Build history of the part. All positions in model axes, mm. A direction names the side the tool comes from. Round coordinates to 2 decimals unless told otherwise and drop trailing zeros. Write each loop counter-clockwise with the first axis right and the second up, starting at its lowest first coordinate (ties: lowest second). Pieces come first, ordered by that corner, then holes. Notation, with made-up numbers: M -4.75,47 L 36.25,47 A15 ccw 36.25,68 Z; hole C 16.5,19 d8. An arc over 180 degrees is marked long. Write item = value, one per line. Start each with the question number.
Q1. Band-saw the part on D-D on y = 0. Write the cut outline in (x, z), plus the area to 3 significant figures.
Q2. Band-saw the part on B-B on y = 9.75. Write the cut outline in (x, z), plus the area to 3 significant figures.
Q3. Tool access for faces 1 (the flat face through (0, 0, 70.202)), 2 (the cylindrical face through (0, -12, 62)), 3 (the flat face through (0, 0, 77.202)): list every direction of +Z, -Z, +X, -X, +Y, -Y with a clear straight run to the whole face (end or side of a thin tool).
Q4. Drop flat-ended pins along their axis: P1, Ø13, axis at y = -2, z = 65, coming from the +X side; P2, Ø7.5, axis at x = -7.5, y = -2, coming from the -Z side; P3, Ø2, axis at x = 10, y = 3, coming from the -Z side; P4, Ø3, axis at x = -2.5, z = 59, coming from the +Y side. Give the stop position or say it passes through.
Q5. Band-saw the part on A-A on z = 59. Write the cut outline in (x, y), plus the area to 3 significant figures.
Q6. Band-saw the part on C-C on x = 0. Write the cut outline in (y, z).
Q7. Pull direction Z, two halves, no side cores. Call faces 4 (the flat face through (8, 0, 74.202)), 5 (the cylindrical face through (0, 12, 62)), 6 (the flat face through (-5, 0, 71)): released by +Z, released by -Z, zero draft, split by the parting line, or undercut.
Q8. Probe L1, parallel to Z at x = 0, y = 7.5; L2, parallel to X at y = -4, z = 70.5; L3, parallel to Y at x = 0, z = 65.5. List the from-to ranges inside material, lowest first.
```python
from build123d import *

# Parameters (mm, degrees)
F1_W          = 15
F1_H          = 25
F3_T          = -3
F4_DEPTH      = 12.0000001006
F4_DEPTH_BACK = 12.0000001006
F5_R          = 2.5
F6_DEPTH      = 5
F7_W          = 10
F7_H          = 7
F8_DEPTH      = 12
F8_DEPTH_BACK = 12


with BuildPart() as f2:
    # F1 (on Front) → F2 (revolve)
    with BuildSketch(Plane.XZ):
        with Locations((7.5, 64.7015325446)):
            Rectangle(F1_W, F1_H)
    revolve(axis=Axis((0, 0, 62.2015325446), (0, 0, 1)))

    # F3
    f3_openings = [f2.faces().sort_by_distance(p)[0] for p in [
        (0, 0, 52.201533),
    ]]
    offset(amount=F3_T, openings=f3_openings)

    # F0 (on Front) → F4 (join, two sides)
    with BuildSketch(Plane.XZ) as f4_sk:
        with BuildLine():
            ThreePointArc((-5, 62.2015325446), (-4.0541927813, 59.2751831307), (-1.5745916432, 57.4559386769))
            ThreePointArc((-1.5745916432, 57.4559386769), (2.9263494138, 58.1473397632), (5, 62.2015325446))
            Line((5, 62.2015325446), (5, 70.2015325446))
            Line((5, 70.2015325446), (-5, 70.2015325446))
            Line((-5, 70.2015325446), (-5, 62.2015325446))
        make_face()
        with BuildLine():
            ThreePointArc((2.5, 62.2015325446), (1.4631747069, 60.1744361539), (-0.7872958216, 59.8287356107))
            ThreePointArc((-0.7872958216, 59.8287356107), (-1.4631747069, 64.2286289352), (2.5, 62.2015325446))
        make_face(mode=Mode.SUBTRACT)
    extrude(amount=-F4_DEPTH)
    extrude(f4_sk.sketch, amount=F4_DEPTH_BACK)

    # F5 (on Front) → F6 (cut, symmetric)
    with BuildSketch(Plane.XZ):
        with BuildLine():
            Line((5, 70.2015325446), (-5, 70.2015325446))
            Line((-5, 70.2015325446), (-5, 62.2015325446))
            ThreePointArc((-5, 62.2015325446), (0, 57.2015325446), (5, 62.2015325446))
            Line((5, 62.2015325446), (5, 70.2015325446))
        make_face()
        with Locations((0, 62.2015325446)):
            Circle(F5_R, mode=Mode.SUBTRACT)
    extrude(amount=F6_DEPTH, both=True, mode=Mode.SUBTRACT)

    # F7 (on Front) → F8 (join, two sides)
    with BuildSketch(Plane.XZ) as f8_sk:
        with Locations((0, 73.7015325446)):
            Rectangle(F7_W, F7_H)
    extrude(amount=F8_DEPTH)
    extrude(f8_sk.sketch, amount=-F8_DEPTH_BACK)


solid = f2.part
```
Conclusion:
q1.outline = M -15,52.2 L -12,52.2 L -12,74.2 L -5,74.2 L -5,70.2 L 5,70.2 L 5,74.2 L 12,74.2 L 12,52.2 L 15,52.2 L 15,77.2 L -15,77.2 Z
q1.area = 262 mm^2
q2.outline = M -11.4,52.2 L -7,52.2 L -7,74.2 L -5,74.2 L -5,62.2 A5 ccw 5,62.2 L 5,74.2 L 7,74.2 L 7,52.2 L 11.4,52.2 L 11.4,77.2 L -11.4,77.2 Z; hole C 0,62.2 d5
q2.area = 402 mm^2
q3.face_1 = -Z
q3.face_2 = none
q3.face_3 = +Z, +X, -X, +Y, -Y
q4.P1 = 15
q4.P2 = 70.2
q4.P3 = 74.2
q4.P4 = 14.97
q5.outline = C 0,0 d30; hole M -3.84,-11.37 L -3.84,-5 L 3.84,-5 L 3.84,-11.37 A12 ccw 3.84,11.37 L 3.84,5 L -3.84,5 L -3.84,11.37 A12 ccw Z
q5.area = 359 mm^2
q6.outline = M -15,52.2 L -12,52.2 L -12,57.2 L -5,57.2 L -5,59.7 L -12,59.7 L -12,64.7 L -5,64.7 L -5,70.2 L 5,70.2 L 5,64.7 L 12,64.7 L 12,59.7 L 5,59.7 L 5,57.2 L 12,57.2 L 12,52.2 L 15,52.2 L 15,77.2 L -15,77.2 Z
q7.face_4 = released by -Z
q7.face_5 = undercut
q7.face_6 = zero draft
q8.L1 = 57.2 to 59.7, 64.7 to 77.2
q8.L2 = -14.46 to -11.31, -5 to 5, 11.31 to 14.46
q8.L3 = -15 to -5, 5 to 15
